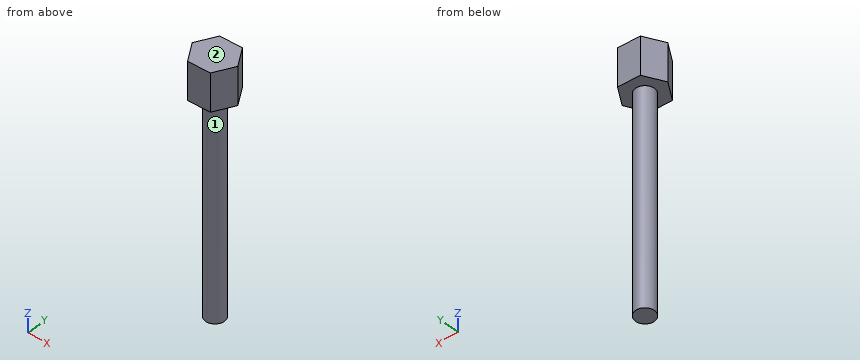
```python
from build123d import *

# Parameters (mm, degrees)
F0_R     = 6.35
F1_DEPTH = 76.2
F2_DEPTH = 67.564
F4_DEPTH = 25.4


with BuildPart() as f1:
    # F0 (on Top) → F1 (new body)
    with BuildSketch(Plane.XY):
        Circle(F0_R)
    extrude(amount=F1_DEPTH)

    # F0 (on Top) → F2 (join)
    with BuildSketch(Plane.XY):
        Circle(F0_R)
    extrude(amount=-F2_DEPTH)

    # F3 (on face) → F4 (join)
    with BuildSketch(Plane.XY.offset(76.2)):
        Polygon((14.64565, 0.747176), (6.675751, 13.057093), (-7.969899, 12.309917), (-14.64565, -0.747176), (-6.675751, -13.057093), (7.969899, -12.309917), align=None)
    extrude(amount=F4_DEPTH)


solid = f1.part
```
Geometry: final body of the model. Coordinates: model frame, mm. Face numbers are marked on the shaded views. A direction names the side the tool comes from. Round coordinates to 2 decimals unless told otherwise and drop trailing zeros. Order: outer loops, then holes, each group sorted by start corner. A loop starts at its lowest first (then second) coordinate and runs counter-clockwise, first axis right, second up. Notation, with made-up numbers: (8, -20) - (54, -20) arc R20 ccw to (54, -6) - close; hole circle Ø11 at (44.5, 17). An arc over 180 degrees is marked (long way). Use CSV: the item, a comma, the result in double quotes. Start each with the question number.
Q1. Section query A-A (y = -3.5). Return loops of the section in (x, z), and give its area (3 significant figures).
Q2. Material intervals for line 1 along Z through (x, y) = (3.75, -7.5); line 2 along X through (y, z) = (-3, 4.5); line 3 along X through (y, z) = (2.75, -19), sorted ascending. Write a range as from..to.
Q3. Section query D-D (x = 12). Return loops of the section in (y, z).
Q4. Section query C-C (z = 7). Return loops of the section in (x, y), and give its area (3 significant figures).
Q5. First-contact query: pin 1 (5 mm diameter, centred on y = 3.5, z = -7, fed in from +X); pin 2 (12 mm diameter, centred on x = -6.5, z = -27, fed in from -Y); pin 3 (6 mm diameter, centred on x = 1.5, z = 84.5, fed in from -Y). Flat tips, straight axial feed; report the tip coordinate or a pass-through.
Q6. Section query B-B (x = 0). Return loops of the section in (y, z).
Q7. Access query for the marked faces 1 and 2. Directions: +Z, -Z, +X, -X, +Y, -Y. A direction counts if a zero-diameter tool reaches every point of the face in a straight line with its end or side. Return the directions, or none.
Result set:
1,outline,"(-12.86, 76.2) - (-5.3, 76.2) - (-5.3, -67.56) - (5.3, -67.56) - (5.3, 76.2) - (12.47, 76.2) - (12.47, 101.6) - (-12.86, 101.6) - close"
1,area,"2,170 mm2"
2,line 1,"z = 76.2..101.6"
2,line 2,"x = -5.6..5.6"
2,line 3,"x = -5.72..5.72"
3,outline,"(-4.43, 76.2) - (4.83, 76.2) - (4.83, 101.6) - (-4.43, 101.6) - close"
4,outline,"circle Ø12.7 at (0, 0)"
4,area,"127 mm2"
5,pin 1,"stops at x = 6.27"
5,pin 2,"stops at y = -6.33"
5,pin 3,"stops at y = -12.79"
6,outline,"(-12.72, 76.2) - (-6.35, 76.2) - (-6.35, -67.56) - (6.35, -67.56) - (6.35, 76.2) - (12.72, 76.2) - (12.72, 101.6) - (-12.72, 101.6) - close"
7,face 1,"-Z"
7,face 2,"+Z, +X, -X, +Y, -Y"
